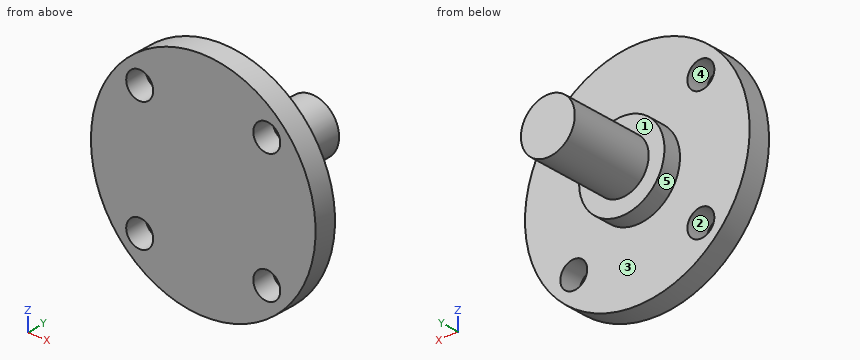
Autodesk Inventor part; units mm, degrees
ref_plane "YZ Plane" through (0, 0, 0) normal (1, 0, 0) x (0, 1, 0)
ref_plane "XZ Plane" through (0, 0, 0) normal (0, 1, 0) x (-1, 0, 0)
ref_plane "XY Plane" through (0, 0, 0) normal (0, 0, 1) x (1, 0, 0)
sketch "Sketch1" plane through (0, 0, 0) normal (0, 1, 0) x (-1, 0, 0)
  circle A0 centre (0, 0) radius 25
  dimension "d0" = 50
extrude "Extrusion1" add sketch "Sketch1" along normal blind 5
sketch "Sketch2" plane through (0, 5, 0) normal (0, 1, 0) x (1, 0, 0)
  line L0 (0, 0) -> (-14.1421, -14.1421) construction
  line L1 (0, 0) -> (20, 0) construction
  point P0 (14.1421, -14.1421)
  point P1 (14.1421, 14.1421)
  point P2 (-14.1421, 14.1421)
  dimension "d3" = 20
  dimension "d4" = 135
  dimension "d7" = 360
hole "Hole1" at (-14.1421, 5, 14.1421) at (14.1421, 5, 14.1421) at (14.1421, 5, -14.1421) at (-14.1421, 5, -14.1421) direction (0, -1, 0) diameter 6 end through all
sketch "Sketch3" plane through (0, 5, 0) normal (0, 1, 0) x (1, 0, 0)
  circle A0 centre (0, 0) radius 9.5
  dimension "d16" = 19
extrude "Extrusion2" add sketch "Sketch3" along normal blind 4
sketch "Sketch4" plane through (0, 9, 0) normal (0, 1, 0) x (1, 0, 0)
  circle A0 centre (0, 0) radius 6
  dimension "d19" = 12
extrude "Extrusion3" add sketch "Sketch4" along normal blind 19
thread "Thread1"
properties part number "PortaMandril"
The model under review builds one solid part; all positions refer to its coordinate system, in mm. Face numbers are marked on the shaded views. A direction names the side the tool comes from. Round coordinates to 2 decimals unless told otherwise and drop trailing zeros. Order: outer loops, then holes, each group sorted by start corner. A loop starts at its lowest first (then second) coordinate and runs counter-clockwise, first axis right, second up.
Item 1: Draft analysis for pull direction Z (two halves, no side actions). For the marked faces 3, 4 and 5, state which applies: released by +Z, released by -Z, zero draft, split by the parting line, or undercut.
Working result:
face 3: zero draft
face 4: undercut
face 5: split by the parting line
Item 2: Machinability: for the marked faces 1 and 2, which of the approach directions +Z, -Z, +X, -X, +Y, -Y give a long, thin tool a straight path to every point of the face, cutting with its end or side? Answer none if there is none.
Working result:
face 1: +Y
face 2: +Y, -Y
Item 3: Add section A-A, the plane z = -12.5. State the section outline as (x, y) points.
Working result:
outline: (-21.65, 0) - (-16.65, 0) - (-16.65, 5) - (-21.65, 5) - close; (-11.63, 0) - (11.63, 0) - (11.63, 5) - (-11.63, 5) - close; (16.65, 0) - (21.65, 0) - (21.65, 5) - (16.65, 5) - close
Item 4: Add section D-D, the plane y = 3.5. State the section outline as (x, z) points, and give its area (3 significant figures).
Working result:
outline: circle Ø50 at (0, 0); hole circle Ø6 at (-14.14, -14.14); hole circle Ø6 at (-14.14, 14.14); hole circle Ø6 at (14.14, -14.14); hole circle Ø6 at (14.14, 14.14)
area: 1,850 mm2
Item 5: Add section C-C, the plane z = 0. State the section outline as (x, y) points.
Working result:
outline: (-25, 0) - (25, 0) - (25, 5) - (9.5, 5) - (9.5, 9) - (6, 9) - (6, 28) - (-6, 28) - (-6, 9) - (-9.5, 9) - (-9.5, 5) - (-25, 5) - close
Item 6: Add section B-B, the plane x = 0. State the section outline as (y, z) points, and give its area (3 significant figures).
Working result:
outline: (0, -25) - (5, -25) - (5, -9.5) - (9, -9.5) - (9, -6) - (28, -6) - (28, 6) - (9, 6) - (9, 9.5) - (5, 9.5) - (5, 25) - (0, 25) - close
area: 554 mm2
Item 7: To check wall thickness, follow probe 1 along Z at (x, y) = (16, 4.5); probe 2 along Z at (x, y) = (-14, 3.25); probe 3 along X at (y, z) = (3.5, -12). State the ranges of each line that lie inside material, in increasing order.
Working result:
probe 1: z = -19.21 to -16.5, -11.79 to 11.79, 16.5 to 19.21
probe 2: z = -20.71 to -17.14, -11.15 to 11.15, 17.14 to 20.71
probe 3: x = -21.93 to -16.24, -12.04 to 12.04, 16.24 to 21.93
Item 8: For pin 1 (2 mm diameter, centred on y = 11, z = -9, fed in from -X); pin 2 (1.5 mm diameter, centred on x = 3.5, y = 24.5, fed in from -Z); pin 3 (8 mm diameter, centred on x = 13.5, z = -2, fed in from +Y); pin 4 (5 mm diameter, centred on y = 15, z = 5, fed in from -X), all flat-tipped, find the tip position at first contact; note any pin that passes through.
Working result:
pin 1: passes through
pin 2: stops at z = -5.33
pin 3: stops at y = 5
pin 4: stops at x = -5.45
